```python
from build123d import *

# Parameters (mm, degrees)
F0_R          = 95
F1_DEPTH      = 25
F1_DEPTH_BACK = 2
F4_DEPTH      = 25
F4_DEPTH_BACK = 2
F5_COUNT      = 6
F8_DEPTH      = 10
F8_DEPTH_BACK = 35
F9_COUNT      = 6
F11_D         = 5
F11_DEPTH     = 13
F11_START     = 2
F11_TIP       = 1.5021515476


with BuildPart() as f1:
    # F0 (on Top) → F1 (new body, two sides)
    with BuildSketch(Plane.XY) as f1_sk:
        Polygon((75, 129.9038105677), (-75, 129.9038105677), (-150, 0), (-75, -129.9038105677), (75, -129.9038105677), (150, 0), align=None)
        Circle(F0_R, mode=Mode.SUBTRACT)
    extrude(amount=-F1_DEPTH)
    extrude(f1_sk.sketch, amount=F1_DEPTH_BACK)


with BuildPart() as f4:
    # F2 (on Top) → F4 (new body, two sides)
    with BuildSketch(Plane.XY) as f4_sk:
        with BuildLine():
            Line((-67.7266746593, 122.6939584625), (-97.9230484541, 70.3923048454))
            ThreePointArc((-97.9230484541, 70.3923048454), (-98.1228492991, 68.8746667552), (-97.1909976466, 67.6602540378))
            Line((-97.1909976466, 67.6602540378), (-68.1009575861, 50.8651115782))
            ThreePointArc((-68.1009575861, 50.8651115782), (-51.4015287339, 67.6969928713), (-30.7025049427, 79.2613158498))
            ThreePointArc((-30.7025049427, 79.2613158498), (-31.770388613, 85.1096644737), (-33.4632679534, 90.8085868892))
            ThreePointArc((-33.4632679534, 90.8085868892), (-34.9064435535, 94.4392315422), (-36.6037204033, 97.9582637535))
            ThreePointArc((-36.6037204033, 97.9582637535), (-48.6270197595, 113.3426973797), (-65.2675230757, 123.5571075336))
            ThreePointArc((-65.2675230757, 123.5571075336), (-66.656996648, 123.5810891624), (-67.7266746593, 122.6939584625))
        make_face()
    extrude(amount=F4_DEPTH)
    extrude(f4_sk.sketch, amount=-F4_DEPTH_BACK)


with BuildPart() as f5_1:
    # F5: instance of F4
    add(f4.part.rotate(Axis((0, 0, -0.1854561269), (0, 0, 1)), 1 * 360 / F5_COUNT))


with BuildPart() as f5_2:
    # F5: instance of F4
    add(f4.part.rotate(Axis((0, 0, -0.1854561269), (0, 0, 1)), 2 * 360 / F5_COUNT))


with BuildPart() as f5_3:
    # F5: instance of F4
    add(f4.part.rotate(Axis((0, 0, -0.1854561269), (0, 0, 1)), 3 * 360 / F5_COUNT))


with BuildPart() as f5_4:
    # F5: instance of F4
    add(f4.part.rotate(Axis((0, 0, -0.1854561269), (0, 0, 1)), 4 * 360 / F5_COUNT))


with BuildPart() as f5_5:
    # F5: instance of F4
    add(f4.part.rotate(Axis((0, 0, -0.1854561269), (0, 0, 1)), 5 * 360 / F5_COUNT))


with BuildPart() as f1_1:
    add(f1.part)

    # F6: cut F5_1, F4, F5_5, F5_4, F5_3, F5_2
    add(f5_1.part, mode=Mode.SUBTRACT)
    add(f4.part, mode=Mode.SUBTRACT)
    add(f5_5.part, mode=Mode.SUBTRACT)
    add(f5_4.part, mode=Mode.SUBTRACT)
    add(f5_3.part, mode=Mode.SUBTRACT)
    add(f5_2.part, mode=Mode.SUBTRACT)


with BuildPart() as f8:
    # F7 (on face) → F8 (new body, two sides)
    with BuildSketch(Plane.XY) as f8_sk:
        with BuildLine():
            ThreePointArc((-66.7217246277, 119.8308093913), (-44.7195832857, 103.2599332678), (-34.5435296861, 77.6643068393))
            ThreePointArc((-34.5435296861, 77.6643068393), (-32.6327882373, 78.4863117484), (-30.7025049427, 79.2613158498))
            ThreePointArc((-30.7025049427, 79.2613158498), (-41.9019572207, 106.1559598637), (-65.2675230757, 123.5571075336))
            ThreePointArc((-65.2675230757, 123.5571075336), (-66.656996648, 123.5810891624), (-67.7266746593, 122.6939584625))
            ThreePointArc((-67.7266746593, 122.6939584625), (-67.8817545517, 121.0315856662), (-66.7217246277, 119.8308093913))
        make_face()
    extrude(amount=F8_DEPTH)
    extrude(f8_sk.sketch, amount=-F8_DEPTH_BACK)


with BuildPart() as f9_1:
    # F9: instance of F8
    add(f8.part.rotate(Axis((0, 0, -0.1854561269), (0, 0, 1)), 1 * 360 / F9_COUNT))


with BuildPart() as f9_2:
    # F9: instance of F8
    add(f8.part.rotate(Axis((0, 0, -0.1854561269), (0, 0, 1)), 2 * 360 / F9_COUNT))


with BuildPart() as f9_3:
    # F9: instance of F8
    add(f8.part.rotate(Axis((0, 0, -0.1854561269), (0, 0, 1)), 3 * 360 / F9_COUNT))


with BuildPart() as f9_4:
    # F9: instance of F8
    add(f8.part.rotate(Axis((0, 0, -0.1854561269), (0, 0, 1)), 4 * 360 / F9_COUNT))


with BuildPart() as f9_5:
    # F9: instance of F8
    add(f8.part.rotate(Axis((0, 0, -0.1854561269), (0, 0, 1)), 5 * 360 / F9_COUNT))


with BuildPart() as f1_2:
    add(f1_1.part)

    # F10: cut F8, F9_5, F9_4, F9_3, F9_2, F9_1
    add(f8.part, mode=Mode.SUBTRACT)
    add(f9_5.part, mode=Mode.SUBTRACT)
    add(f9_4.part, mode=Mode.SUBTRACT)
    add(f9_3.part, mode=Mode.SUBTRACT)
    add(f9_2.part, mode=Mode.SUBTRACT)
    add(f9_1.part, mode=Mode.SUBTRACT)

    # F11
    # its depths count from where the whole tool has entered the part; down to there all is cleared
    with Locations(Plane.XY.offset(-F11_START)):
        with Locations((20, 110), (105.2627944163, 37.6794919243), (85.2627944163, -72.3205080757), (-20, -110), (-105.2627944163, -37.6794919243), (-85.2627944163, 72.3205080757)):
            Hole(F11_D / 2, depth=F11_DEPTH)
            with Locations((0, 0, -(F11_DEPTH + F11_TIP / 2))):  # 118° drill point
                Cone(0, F11_D / 2, F11_TIP, mode=Mode.SUBTRACT)


solid = f1_2.part
```
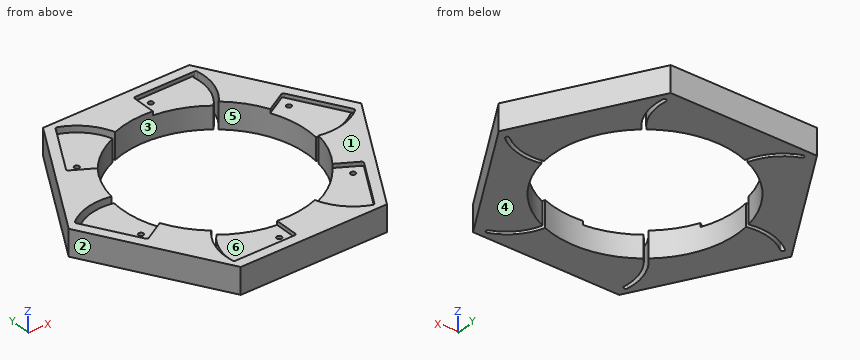
For this review, take the finished solid that the model builds, in its own axes (mm). Face numbers are marked on the shaded views. A direction names the side the tool comes from. Round coordinates to 2 decimals unless told otherwise and drop trailing zeros. Write each loop counter-clockwise with the first axis right and the second up, starting at its lowest first coordinate (ties: lowest second). Pieces come first, ordered by that corner, then holes.
1) Mouldability with a two-part tool opening along Y and no side actions: class the marked faces 1, 2 and 3 as +Y half, -Y half, draft (parallel to the pull), parting line (faces both ways), or undercut.
Answer below:
face 1: draft
face 2: -Y half
face 3: undercut
2) Take a section at D-D on x = 53. Give the boundary of the cut face in (y, z).
Answer below:
outline: (-129.9, -25) - (-116.86, -25) - (-116.86, 2) - (-129.9, 2) - close; (-111.82, -25) - (-78.84, -25) - (-78.84, -2) - (-111.82, -2) - close; (78.84, -25) - (129.9, -25) - (129.9, 2) - (120, 2) - (120, -2) - (78.84, -2) - close
3) Insertion check: pin 1 Ø6 at (x, z) = (-105.5, -8.5) entering from +Y; pin 2 Ø10 at (y, z) = (72, -1) entering from +X; pin 3 Ø8 at (y, z) = (1, -3) entering from -X. Each pin has a flat end and moves straight along its axis. Give the tip position at first contact, or say it passes through.
Answer below:
pin 1: stops at y = 82.27
pin 2: stops at x = 111.32
pin 3: stops at x = -150
4) Machinability: for the marked faces 4, 5 and 6, which of the approach directions +Z, -Z, +X, -X, +Y, -Y give a long, thin tool a straight path to every point of the face, cutting with its end or side? Answer none if there is none.
Answer below:
face 4: -Z, +X, -X, +Y, -Y
face 5: +Z, -Z
face 6: +Z
5) Take a section at A-A on y = -44.5. Give the boundary of the cut face in (x, z), then the cut area to 3 significant figures.
Answer below:
outline: (-124.31, -25) - (-83.93, -25) - (-83.93, 2) - (-97.08, 2) - (-97.08, -2) - (-112.87, -2) - (-112.87, 2) - (-124.31, 2) - close; (83.93, -25) - (124.31, -25) - (124.31, 2) - (83.93, 2) - close
area: 2,120 mm2
6) Take a section at B-B on x = 129.5. Give the boundary of the cut face in (y, z).
Answer below:
outline: (-35.51, -25) - (-11.69, -25) - (-11.69, 2) - (-35.51, 2) - close; (-7.19, -25) - (35.51, -25) - (35.51, 2) - (15.7, 2) - (15.7, -2) - (-7.19, -2) - close
7) For line 1 along Y through (x, z) = (-1, -13.5); line 2 along X through (y, z) = (110, -11.75); line 3 along X through (y, z) = (-115.5, -22), list the stretches that pass through material, from the lowest coordinate up.
Answer below:
line 1: y = -129.9 to -94.99, 94.99 to 129.9
line 2: x = -86.49 to -50.89, -45.2 to 17.5, 22.5 to 71, 75 to 86.49
line 3: x = -83.32 to -74.72, -70.7 to 51.2, 58.12 to 83.32
